Read the model definition and answer for the solid it produces. Units are mm, in the model's axes. Face numbers are marked on the shaded views. A direction names the side the tool comes from. Coordinates: 2 decimals unless noted, no trailing zeros. Write each loop counter-clockwise with the first axis right and the second up, starting at its lowest first coordinate (ties: lowest second). Pieces come first, ordered by that corner, then holes. Notation, with made-up numbers: M 23.5,7 L 29.5,7 A6 cw 29.5,11 Z; hole C -3,-10.5 d11. An arc over 180 degrees is marked long. Use a Markdown table: item, result. Add a question column.
from build123d import *

# Parameters (mm, degrees)
ESQUISSE1_R        = 37.50000000000001
BOSS_EXTRU_1_DEPTH = 2
ESQUISSE2_W        = 30.000000000000004
ESQUISSE2_H        = 1.4999999999999964
ESQUISSE2_W_2      = 1.5
ESQUISSE2_H_2      = 10
EXTRU_MINCE1_DEPTH = 4.7
ESQUISSE5_W        = 16
ESQUISSE5_H        = 2.0000000000000036
BOSS_EXTRU_3_DEPTH = 1
CONG_5_R           = 0.5
CONG_6_R           = 0.5
CONG_1_R           = 4.6
CONG_2_R           = 4.6
EXTRU_MINCE2_DEPTH = 6.5
BOSS_EXTRU_2_DEPTH = 1
BOSS_EXTRU_5_DEPTH = 1
BOSS_EXTRU_4_DEPTH = 8.5
CHANFREIN1_SIZE    = 1
CONG_7_R           = 4


# Some blends are built 0.0001 mm under size
with BuildPart() as part:
    # Esquisse1 → Boss.-Extru.1 (new body)
    with BuildSketch(Plane.XY):
        Circle(ESQUISSE1_R)
        with BuildLine():
            Line((-21.999999999999996, -18.999999999999996), (22.000000000000004, -18.999999999999996))
            ThreePointArc((22.000000000000004, -18.999999999999996), (22.353553390593277, -18.85355339059327), (22.500000000000004, -18.499999999999996))
            Line((22.500000000000004, -18.499999999999996), (22.500000000000004, 18.500000000000004))
            ThreePointArc((22.500000000000004, 18.500000000000004), (22.353553390593277, 18.853553390593277), (22.000000000000004, 19.000000000000004))
            Line((22.000000000000004, 19.000000000000004), (-21.999999999999996, 19.000000000000004))
            ThreePointArc((-21.999999999999996, 19.000000000000004), (-22.35355339059327, 18.853553390593277), (-22.499999999999996, 18.500000000000004))
            Line((-22.499999999999996, 18.500000000000004), (-22.499999999999996, -18.499999999999996))
            ThreePointArc((-22.499999999999996, -18.499999999999996), (-22.35355339059327, -18.85355339059327), (-21.999999999999996, -18.999999999999996))
        make_face(mode=Mode.SUBTRACT)
    extrude(amount=BOSS_EXTRU_1_DEPTH)

    # Esquisse2 → Extru.-Mince1 (add)
    with BuildSketch(Plane.XY.offset(2)):
        with Locations((0, 22.4)):
            Rectangle(ESQUISSE2_W, ESQUISSE2_H)
        with Locations((31.05, 0)):
            Rectangle(ESQUISSE2_W_2, ESQUISSE2_H_2)
        with Locations((-31.05, 0)):
            Rectangle(ESQUISSE2_W_2, ESQUISSE2_H_2)
        with Locations((0, -22.4)):
            Rectangle(ESQUISSE2_W, ESQUISSE2_H)
    extrude(amount=EXTRU_MINCE1_DEPTH)

    # Esquisse5 → Boss.-Extru.3 (add)
    with BuildSketch(Plane.XY.offset(6.7)):
        with Locations((0, 22.15)):
            Rectangle(ESQUISSE5_W, ESQUISSE5_H)
        with Locations((0, -22.15)):
            Rectangle(ESQUISSE5_W, ESQUISSE5_H)
    extrude(amount=BOSS_EXTRU_3_DEPTH)

    # Congé5
    # the kernel refuses this fillet: 0.5 mm, written as the material it takes off along each edge
    with BuildSketch(Plane(origin=(9.25, 21.15, 6.7), x_dir=(0, 1, 0), z_dir=(-1, 0, 0))) as cong_5_piece_1:
        with BuildLine():
            CenterArc((CONG_5_R, -CONG_5_R), CONG_5_R, 90, 90)
            Line((0, -CONG_5_R), (0, 0))
            Line((0, 0), (CONG_5_R, 0))
        make_face()
    extrude(amount=18.5, mode=Mode.SUBTRACT)
    with BuildSketch(Plane(origin=(9.25, 21.15, 7.7), x_dir=(0, 0, -1), z_dir=(-1, 0, 0))) as cong_5_piece_2:
        with BuildLine():
            CenterArc((CONG_5_R, -CONG_5_R), CONG_5_R, 90, 90)
            Line((0, -CONG_5_R), (0, 0))
            Line((0, 0), (CONG_5_R, 0))
        make_face()
    extrude(amount=18.5, mode=Mode.SUBTRACT)

    # Congé6
    # the kernel refuses this fillet: 0.5 mm, written as the material it takes off along each edge
    with BuildSketch(Plane(origin=(9.25, -21.15, 6.7), x_dir=(0, -1, 0), z_dir=(-1, 0, 0))) as cong_6_piece_1:
        with BuildLine():
            CenterArc((CONG_6_R, CONG_6_R), CONG_6_R, 180, 90)
            Line((0, CONG_6_R), (0, 0))
            Line((0, 0), (CONG_6_R, 0))
        make_face()
    extrude(amount=18.5, mode=Mode.SUBTRACT)
    with BuildSketch(Plane(origin=(9.25, -21.15, 7.7), x_dir=(0, -1, 0), z_dir=(-1, 0, 0))) as cong_6_piece_2:
        with BuildLine():
            CenterArc((CONG_6_R, -CONG_6_R), CONG_6_R, 90, 90)
            Line((0, -CONG_6_R), (0, 0))
            Line((0, 0), (CONG_6_R, 0))
        make_face()
    extrude(amount=18.5, mode=Mode.SUBTRACT)

    # Congé1
    cong_1_edges = [part.edges().sort_by_distance(p)[0] for p in [
        (-15, 22.4, 2),
        (15, 22.4, 2),
        (31.05, -5, 2),
        (31.05, 5, 2),
        (-31.05, -5, 2),
        (-31.05, 5, 2),
        (-15, -22.4, 2),
        (15, -22.4, 2),
    ]]
    fillet(cong_1_edges, radius=CONG_1_R)

    # Congé2
    cong_2_edges = [part.edges().sort_by_distance(p)[0] for p in [
        (15, 22.4, 6.7),
        (31.05, 5, 6.7),
        (31.05, -5, 6.7),
        (15, -22.4, 6.7),
        (-15, -22.4, 6.7),
        (-31.05, 5, 6.7),
        (-31.05, -5, 6.7),
        (-15, 22.4, 6.7),
    ]]
    fillet(cong_2_edges, radius=CONG_2_R)

    # Esquisse3 → Extru.-Mince2 (add)
    with BuildSketch(Plane.XY.offset(2)):
        with BuildLine():
            ThreePointArc((-32.80000000000001, 10.369185117452545), (-34.4, 4.21e-15), (-32.80000000000001, -10.369185117452545))
            Line((-32.80000000000001, -10.369185117452545), (-31.84651162790699, -10.0677553175266))
            ThreePointArc((-31.84651162790699, -10.0677553175266), (-33.4, -4.09e-15), (-31.84651162790699, 10.0677553175266))
            Line((-31.84651162790699, 10.0677553175266), (-32.80000000000001, 10.369185117452545))
        make_face()
        with BuildLine():
            ThreePointArc((-19.772139489696098, -28.150000000000002), (2.11e-15, -34.4), (19.772139489696098, -28.150000000000002))
            Line((19.772139489696098, -28.150000000000002), (19.197367992902606, -27.33168604651163))
            ThreePointArc((19.197367992902606, -27.33168604651163), (2.05e-15, -33.4), (-19.197367992902606, -27.33168604651163))
            Line((-19.197367992902606, -27.33168604651163), (-19.772139489696098, -28.150000000000002))
        make_face()
        with BuildLine():
            ThreePointArc((32.80000000000001, -10.369185117452545), (34.4, 0), (32.80000000000001, 10.369185117452545))
            Line((32.80000000000001, 10.369185117452545), (31.84651162790699, 10.0677553175266))
            ThreePointArc((31.84651162790699, 10.0677553175266), (33.4, 0), (31.84651162790699, -10.0677553175266))
            Line((31.84651162790699, -10.0677553175266), (32.80000000000001, -10.369185117452545))
        make_face()
        with BuildLine():
            ThreePointArc((19.772139489696105, 28.15), (2.11e-15, 34.4), (-19.772139489696105, 28.15))
            Line((-19.772139489696105, 28.15), (-19.197367992902613, 27.331686046511628))
            ThreePointArc((-19.197367992902613, 27.331686046511628), (-5.37e-15, 33.4), (19.197367992902613, 27.331686046511628))
            Line((19.197367992902613, 27.331686046511628), (19.772139489696105, 28.15))
        make_face()
    extrude(amount=EXTRU_MINCE2_DEPTH)

    # Esquisse4 → Boss.-Extru.2 (add)
    with BuildSketch(Plane.XY.offset(8.5)):
        with BuildLine():
            Line((-19.197367992902617, 27.331686046511624), (-20.3469109864896, 28.96831395348837))
            ThreePointArc((-20.3469109864896, 28.96831395348837), (-5.69e-15, 35.400000000000006), (20.346910986489593, 28.968313953488376))
            Line((20.346910986489593, 28.968313953488376), (19.19736799290261, 27.331686046511624))
            ThreePointArc((19.19736799290261, 27.331686046511624), (2.05e-15, 33.4), (-19.197367992902617, 27.331686046511624))
        make_face()
        with BuildLine():
            Line((33.75348837209304, 10.67061491737849), (31.84651162790699, 10.067755317526597))
            ThreePointArc((31.84651162790699, 10.067755317526597), (33.4, -3.71e-15), (31.846511627906985, -10.067755317526604))
            Line((31.846511627906985, -10.067755317526604), (33.753488372093045, -10.670614917378492))
            ThreePointArc((33.753488372093045, -10.670614917378492), (35.40000000000001, 0), (33.75348837209304, 10.67061491737849))
        make_face()
        with BuildLine():
            Line((19.197367992902603, -27.331686046511635), (20.346910986489593, -28.968313953488376))
            ThreePointArc((20.346910986489593, -28.968313953488376), (1.003e-14, -35.4), (-20.34691098648957, -28.96831395348839))
            Line((-20.34691098648957, -28.96831395348839), (-19.197367992902635, -27.33168604651161))
            ThreePointArc((-19.197367992902635, -27.33168604651161), (-2.762e-14, -33.4), (19.197367992902603, -27.331686046511635))
        make_face()
        with BuildLine():
            Line((-31.846511627906985, -10.067755317526593), (-33.75348837209304, -10.670614917378492))
            ThreePointArc((-33.75348837209304, -10.670614917378492), (-35.40000000000001, 4.34e-15), (-33.753488372093045, 10.67061491737849))
            Line((-33.753488372093045, 10.67061491737849), (-31.846511627906985, 10.067755317526604))
            ThreePointArc((-31.846511627906985, 10.067755317526604), (-33.4, 4.09e-15), (-31.846511627906985, -10.067755317526593))
        make_face()
    extrude(amount=BOSS_EXTRU_2_DEPTH)

    # Esquisse8 → Boss.-Extru.5 (add)
    with BuildSketch(Plane.XY.offset(9.500000000000002)):
        with BuildLine():
            Line((20.34691098648959, -28.96831395348837), (18.622596496109104, -26.513372093023264))
            ThreePointArc((18.622596496109104, -26.513372093023264), (-4.118e-14, -32.4), (-18.622596496109168, -26.513372093023218))
            Line((-18.622596496109168, -26.513372093023218), (-20.34691098648957, -28.96831395348839))
            ThreePointArc((-20.34691098648957, -28.96831395348839), (1.003e-14, -35.4), (20.34691098648959, -28.96831395348837))
        make_face()
        with BuildLine():
            Line((-20.346910986489604, 28.968313953488373), (-18.622596496109125, 26.51337209302325))
            ThreePointArc((-18.622596496109125, 26.51337209302325), (1.98e-15, 32.4), (18.622596496109125, 26.513372093023253))
            Line((18.622596496109125, 26.513372093023253), (20.346910986489593, 28.968313953488384))
            ThreePointArc((20.346910986489593, 28.968313953488384), (-1.355e-14, 35.40000000000001), (-20.346910986489604, 28.968313953488373))
        make_face()
    extrude(amount=BOSS_EXTRU_5_DEPTH)

    # Esquisse7 → Boss.-Extru.4 (add)
    with BuildSketch(Plane.XY.offset(2)):
        with BuildLine():
            Line((0.9999999999999993, 36.400000000000006), (1.0000000000000009, 31.400000000000006))
            ThreePointArc((1.0000000000000009, 31.400000000000006), (-1.8e-16, 30.400000000000006), (-0.9999999999999996, 31.400000000000006))
            Line((-0.9999999999999996, 31.400000000000006), (-1.000000000000001, 36.400000000000006))
            ThreePointArc((-1.000000000000001, 36.400000000000006), (-1.47e-15, 37.400000000000006), (0.9999999999999993, 36.400000000000006))
        make_face()
    extrude(amount=BOSS_EXTRU_4_DEPTH)

    # Chanfrein1
    chanfrein1_edges = [part.edges().sort_by_distance(p)[0] for p in [
        (10.843924173071517, 32.64612241183745, 8.5),
        (-3.55e-15, -34.39999999999999, 8.5),
        (34.400000000000006, 4e-15, 8.5),
        (-34.4, -8.9e-16, 8.5),
        (-10.542492654739178, 31.692520389277497, 9.5),
        (-1.776e-14, -33.39999999999999, 9.5),
        (10.542492654739181, 31.692520389277497, 9.5),
        (-10.843924173071517, 32.64612241183745, 8.5),
    ]]
    chamfer(chanfrein1_edges, length=CHANFREIN1_SIZE - 0.0001)  # a hair under: the kernel refuses the full size

    # Congé7
    # the kernel refuses this fillet: 4 mm, written as the material it adds along each edge
    with BuildSketch(Plane(origin=(8, -23.150000000000002, 6.7), x_dir=(1, 0, -3.4e-16), z_dir=(0, 1, 0)), Plane(origin=(-8, -21.65, 6.7), x_dir=(-1, 0, -3.4e-16), z_dir=(0, -1, 0))) as cong_7_piece_1:
        with BuildLine():
            CenterArc((2.645751311064592, -4), CONG_7_R, 89.99999999999999, 41.4096221092709)
            Line((-3.4e-16, -1.0000000000000009), (0, 0))
            Line((0, 0), (2.6457513110645934, 0))
        make_face()
    extrude(amount=1.5000000000000036)
    with BuildSketch(Plane(origin=(-8, 21.65, 6.7), x_dir=(0, 0, 1), z_dir=(0, 1, 0))) as cong_7_piece_2:
        with BuildLine():
            CenterArc((3.999999999999999, -2.6457513110645934), CONG_7_R, 138.5903778907291, 41.40962210927091)
            Line((-8.9e-16, -2.6457513110645934), (0, 0))
            Line((0, 0), (1.0000000000000009, 0))
        make_face()
    extrude(amount=1.5000000000000036)
    with BuildSketch(Plane(origin=(8, 23.150000000000002, 6.7), x_dir=(1, 0, -3.4e-16), z_dir=(0, -1, 0))) as cong_7_piece_3:
        with BuildLine():
            CenterArc((2.645751311064592, 4), CONG_7_R, 228.59037789072912, 41.40962210927091)
            Line((-3.4e-16, 1.0000000000000009), (0, 0))
            Line((0, 0), (2.6457513110645934, 0))
        make_face()
    extrude(amount=1.5000000000000036)


solid = part.part
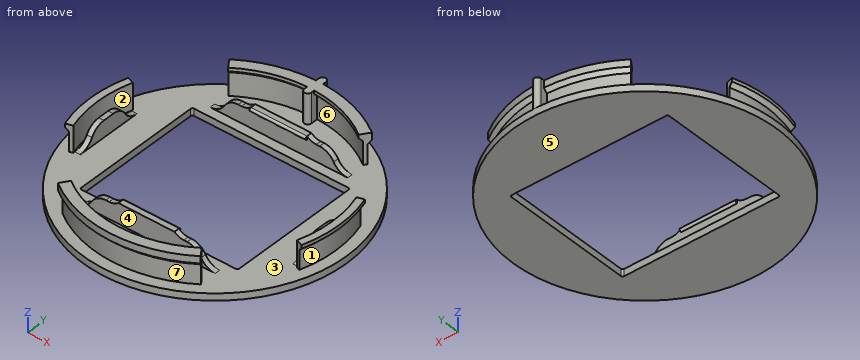
Item 1: Consider probe 1 along Y at (x, z) = (13, 2.5); probe 2 along Y at (x, z) = (-7.5, 7.5); probe 3 along X at (y, z) = (-4, 2.75). Determine where each line is inside the solid, lowest interval first.
Item 2: Determine the mould class of the marked faces 5, 6 and 7 for opening direction X: pulls with the +X half, pulls with the -X half, needs draft (parallel to the pull), parting line crosses it, or undercut.
Item 3: Find section B-B on y = 25.5. Give the vertices of the cut face in (x, z), then the cut area to 3 significant figures.
Item 4: For the marked faces 1, 2, 3 and 4, determine the directions among +Z, -Z, +X, -X, +Y, -Y from which every point of the face is accessible in a straight line to the end or side of a thin tool.
Item 5: Find section A-A on z = 3.25. Count the separate pieces of the cut face and the enclosed holes in it, then the cut area to 3 significant figures.
Item 6: Each of these flat-tipped pins is pushed along its axis until it touches: pin 1 (6 mm diameter, centred on x = 19, z = 3, fed in from -Y); pin 2 (0.5 mm diameter, centred on x = 11.5, y = -22.5, fed in from +Z); pin 3 (1.8 mm diameter, centred on x = -33, y = 2.5, fed in from +Z). Where does it stop, or does it pass through?
Geometry says:
| question | item | result |
|---|---|---|
| 1 | probe 1 | y = -31.85 to -30.77, -23.15 to -21.65, 21.65 to 23.15, 30.77 to 31.85 |
| 1 | probe 2 | y = -33.57 to -32.55, -23.15 to -21.25, 21.25 to 23.15, 32.55 to 33.57 |
| 1 | probe 3 | x = -34.17 to -33.16, -31.8 to -30.3, 30.3 to 31.8, 33.16 to 34.17 |
| 2 | face 5 | needs draft |
| 2 | face 6 | undercut |
| 2 | face 7 | parting line crosses it |
| 3 | outline | M -27.5,0 L 27.5,0 L 27.5,2 L -27.5,2 Z |
| 3 | area | 110 mm2 |
| 4 | face 1 | +X |
| 4 | face 2 | +Z |
| 4 | face 3 | none |
| 4 | face 4 | +Z, +X, -X |
| 5 | separate pieces | 8 |
| 5 | enclosed holes | 0 |
| 5 | area | 273 mm2 |
| 6 | pin 1 | stops at y = -33.83 |
| 6 | pin 2 | stops at z = 6.7 |
| 6 | pin 3 | stops at z = 9.5 |
